Geometry: final body of the model. Coordinates: model frame, mm. Face numbers are marked on the shaded views. Give positions to 0.01 mm unless a question says otherwise; leave off trailing zeros. Write each loop counter-clockwise with the first axis right and the second up, starting at its lowest first coordinate (ties: lowest second). Pieces come first, ordered by that corner, then holes. Notation, with made-up numbers: (38, -32.5) -> (69, -32.5) arc R24 ccw to (69, 3.5) -> close; hole circle Ø10 at (18, -15.5). An arc over 180 degrees is marked (long way). Answer in a Markdown table with one row per item. Add a question column.
Item 1: Section query A-A on x = 0. Output: boundary loops of the cut face in (y, z), plus the area to 3 significant figures.
Item 2: First-contact query: P1, Ø3, axis at y = 18.5, z = 2, coming from the -X side; P2, Ø1.5, axis at y = 30, z = 3.5, coming from the +X side; P3, Ø1.5, axis at x = 1, z = 2.5, coming from the +Y side; P4, Ø2.5, axis at y = 29.5, z = 4.5, coming from the -X side. Flat tips, straight axial feed; report the tip coordinate or a pass-through.
Item 3: Draft query along X for the marked faces 1 and 2. Return one class per face: +X half, -X half, draft (parallel to the pull), parting line (faces both ways), or undercut.
Item 4: Section query C-C on y = 6. Output: boundary loops of the cut face in (x, z), plus the area to 3 significant figures.
Item 5: Section query B-B on z = 3. Output: boundary loops of the cut face in (x, y), plus the area to 3 significant figures.
Item 6: Material intervals for probe 1 along Z at (x, y) = (-2.5, -26.5); probe 2 along Y at (x, z) = (-1.5, 2.25); probe 3 along Z at (x, y) = (-2, -2.5), sorted ascending. Write a range as from..to.
```python
from build123d import *

# Parameters (mm, degrees)
BOSS_EXTRUDE1_DEPTH     = 1
CUT_EXTRUDE2_DEPTH      = 35.5
CUT_EXTRUDE2_DEPTH_BACK = 33.5
SKETCH3_W               = 5
SKETCH3_H               = 3
BOSS_EXTRUDE2_DEPTH     = 5


with BuildPart() as part:
    # Sketch1 → Boss-Extrude1 (new body, symmetric)
    with BuildSketch(Plane.XY):
        with BuildLine():
            Line((-2.7, 32.5), (-2.7, -32.5))
            ThreePointArc((-2.7, -32.5), (0, -29.8), (2.7, -32.5))
            Line((2.7, -32.5), (2.7, 32.5))
            Line((2.7, 32.5), (-2.7, 32.5))
        make_face()
        Polygon((4.7, -32.5), (2.7, -32.5), (2.7, 32.5), (-2.7, 32.5), (-2.7, -32.5), (-4.7, -32.5), (-4.7, 34.5), (4.7, 34.5), align=None)
    extrude(amount=BOSS_EXTRUDE1_DEPTH, both=True)

    # Sketch2 → Cut-Extrude2 (cut, two sides)
    with BuildSketch(Plane(origin=(0, 0, 0), x_dir=(1, 0, 0), z_dir=(0, 1, 0))) as cut_extrude2_sk:
        with BuildLine():
            ThreePointArc((-4.7, 1), (0, 0.805897581), (4.7, 1))
            Line((4.7, 1), (-4.7, 1))
        make_face()
        with BuildLine():
            Line((-4.7, 1), (4.7, 1))
            ThreePointArc((4.7, 1), (41.93387652, 19.198255851), (57, 57.805897581))
            ThreePointArc((57, 57.805897581), (-38.607641731, 99.739774101), (-4.7, 1))
        make_face()
    extrude(amount=CUT_EXTRUDE2_DEPTH, mode=Mode.SUBTRACT)
    extrude(cut_extrude2_sk.sketch, amount=-CUT_EXTRUDE2_DEPTH_BACK, mode=Mode.SUBTRACT)

    # Sketch3 → Boss-Extrude2 (add)
    with BuildSketch(Plane.XY.offset(1)):
        with Locations((0, 29.5)):
            Rectangle(SKETCH3_W, SKETCH3_H)
    extrude(amount=BOSS_EXTRUDE2_DEPTH)


solid = part.part
```
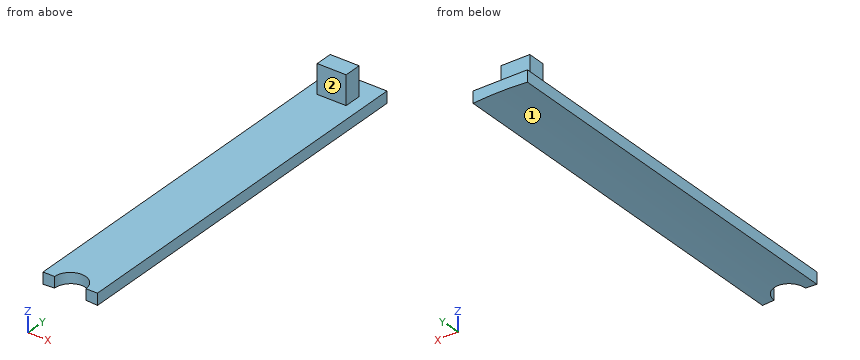
Findings below:
| question | item | result |
|---|---|---|
| 1 | outline | (-29.8, -0.81) -> (34.5, -0.81) -> (34.5, 1) -> (31, 1) -> (31, 6) -> (28, 6) -> (28, 1) -> (-29.8, 1) -> close |
| 1 | area | 131 mm^2 |
| 2 | P1 | stops at x = -4.7 |
| 2 | P2 | stops at x = 2.5 |
| 2 | P3 | stops at y = 31 |
| 2 | P4 | stops at x = -2.5 |
| 3 | face 1 | undercut |
| 3 | face 2 | draft |
| 4 | outline | (-4.7, -1) arc R57 cw to (4.7, -1) -> (4.7, 1) -> (-4.7, 1) -> close |
| 4 | area | 17.6 mm^2 |
| 5 | outline | (-2.5, 28) -> (2.5, 28) -> (2.5, 31) -> (-2.5, 31) -> close |
| 5 | area | 15.0 mm^2 |
| 6 | probe 1 | z = -0.86..1 |
| 6 | probe 2 | y = 28..31 |
| 6 | probe 3 | z = -0.84..1 |
